```python
from build123d import *

# Parameters (mm, degrees)
SKETCH1_W           = 62.16
SKETCH1_H           = 32.16
SKETCH1_W_2         = 59.16
SKETCH1_H_2         = 29.16
BOSS_EXTRUDE1_DEPTH = 19
SKETCH2_W           = 62.16
SKETCH2_H           = 32.16
BOSS_EXTRUDE2_DEPTH = 1
BOSS_EXTRUDE3_DEPTH = 5
CUT_EXTRUDE4_DEPTH  = 2
CUT_EXTRUDE2_DEPTH  = 33.16
CUT_EXTRUDE3_DEPTH  = 63.16
SKETCH9_W           = 7
SKETCH9_H           = 8.75
CUT_EXTRUDE5_DEPTH  = 63.16


with BuildPart() as part:
    # Sketch1 → Boss-Extrude1 (new body)
    with BuildSketch(Plane.XY):
        Rectangle(SKETCH1_W, SKETCH1_H)
        Rectangle(SKETCH1_W_2, SKETCH1_H_2, mode=Mode.SUBTRACT)
    extrude(amount=BOSS_EXTRUDE1_DEPTH)

    # Sketch2 → Boss-Extrude2 (add)
    with BuildSketch(Plane.XY.offset(19)):
        Rectangle(SKETCH2_W, SKETCH2_H)
    extrude(amount=BOSS_EXTRUDE2_DEPTH)

    # Sketch3 → Boss-Extrude3 (add)
    with BuildSketch(Plane(origin=(0, 0, 0), x_dir=(-1, 0, 0), z_dir=(0, 0, -1))):
        Polygon((-31.08, -16.08), (31.08, -16.08), (31.08, 16.08), (9, 16.08), (-9, 16.08), (-31.08, 16.08), align=None)
        Polygon((29.58, -14.58), (-29.58, -14.58), (-29.58, 14.58), (-9, 14.58), (9, 14.58), (29.58, 14.58), align=None, mode=Mode.SUBTRACT)
    extrude(amount=BOSS_EXTRUDE3_DEPTH)

    # Sketch8 → Cut-Extrude4 (cut, through all)
    with BuildSketch(Plane(origin=(0, 0, 19), x_dir=(-1, 0, 0), z_dir=(0, 0, -1))):
        with BuildLine():
            Line((12, 6.5), (22, 6.5))
            ThreePointArc((22, 6.5), (24, 8.5), (22, 10.5))
            Line((22, 10.5), (12, 10.5))
            ThreePointArc((12, 10.5), (10, 8.5), (12, 6.5))
        make_face()
        with BuildLine():
            Line((12, -2), (22, -2))
            ThreePointArc((22, -2), (24, 0), (22, 2))
            Line((22, 2), (12, 2))
            ThreePointArc((12, 2), (10, 0), (12, -2))
        make_face()
        with BuildLine():
            Line((12, -10.5), (22, -10.5))
            ThreePointArc((22, -10.5), (24, -8.5), (22, -6.5))
            Line((22, -6.5), (12, -6.5))
            ThreePointArc((12, -6.5), (10, -8.5), (12, -10.5))
        make_face()
        with BuildLine():
            Line((-5, -10.5), (5, -10.5))
            ThreePointArc((5, -10.5), (7, -8.5), (5, -6.5))
            Line((5, -6.5), (-5, -6.5))
            ThreePointArc((-5, -6.5), (-7, -8.5), (-5, -10.5))
        make_face()
        with BuildLine():
            Line((-22, -10.5), (-12, -10.5))
            ThreePointArc((-12, -10.5), (-10, -8.5), (-12, -6.5))
            Line((-12, -6.5), (-22, -6.5))
            ThreePointArc((-22, -6.5), (-24, -8.5), (-22, -10.5))
        make_face()
        with BuildLine():
            Line((-22, -2), (-12, -2))
            ThreePointArc((-12, -2), (-10, 0), (-12, 2))
            Line((-12, 2), (-22, 2))
            ThreePointArc((-22, 2), (-24, 0), (-22, -2))
        make_face()
        with BuildLine():
            Line((-5, 6.5), (5, 6.5))
            ThreePointArc((5, 6.5), (7, 8.5), (5, 10.5))
            Line((5, 10.5), (-5, 10.5))
            ThreePointArc((-5, 10.5), (-7, 8.5), (-5, 6.5))
        make_face()
        with BuildLine():
            Line((-22, 6.5), (-12, 6.5))
            ThreePointArc((-12, 6.5), (-10, 8.5), (-12, 10.5))
            Line((-12, 10.5), (-22, 10.5))
            ThreePointArc((-22, 10.5), (-24, 8.5), (-22, 6.5))
        make_face()
        with BuildLine():
            Line((-5, -2), (5, -2))
            ThreePointArc((5, -2), (7, 0), (5, 2))
            Line((5, 2), (-5, 2))
            ThreePointArc((-5, 2), (-7, 0), (-5, -2))
        make_face()
    extrude(amount=-CUT_EXTRUDE4_DEPTH, mode=Mode.SUBTRACT)

    # Sketch5 → Cut-Extrude2 (cut, through all)
    with BuildSketch(Plane(origin=(-15, 16.08, 0), x_dir=(1, 0, 0), z_dir=(0, -1, 0))):
        with BuildLine():
            Line((-9.5, 4), (0.5, 4))
            ThreePointArc((0.5, 4), (2.5, 2), (0.5, 0))
            Line((0.5, 0), (-9.5, 0))
            ThreePointArc((-9.5, 0), (-11.5, 2), (-9.5, 4))
        make_face()
        with BuildLine():
            Line((10, -32.734958022), (20, -32.734958022))
            ThreePointArc((20, -32.734958022), (22, -30.734958022), (20, -28.734958022))
            Line((20, -28.734958022), (10, -28.734958022))
            ThreePointArc((10, -28.734958022), (8, -30.734958022), (10, -32.734958022))
        make_face()
        with BuildLine():
            Line((29.5, -65.469916045), (39.5, -65.469916045))
            ThreePointArc((39.5, -65.469916045), (41.5, -63.469916045), (39.5, -61.469916045))
            Line((39.5, -61.469916045), (29.5, -61.469916045))
            ThreePointArc((29.5, -61.469916045), (27.5, -63.469916045), (29.5, -65.469916045))
        make_face()
        with BuildLine():
            Line((10, -21.734958022), (20, -21.734958022))
            ThreePointArc((20, -21.734958022), (22, -19.734958022), (20, -17.734958022))
            Line((20, -17.734958022), (10, -17.734958022))
            ThreePointArc((10, -17.734958022), (8, -19.734958022), (10, -21.734958022))
        make_face()
        with BuildLine():
            Line((29.5, -54.469916045), (39.5, -54.469916045))
            ThreePointArc((39.5, -54.469916045), (41.5, -52.469916045), (39.5, -50.469916045))
            Line((39.5, -50.469916045), (29.5, -50.469916045))
            ThreePointArc((29.5, -50.469916045), (27.5, -52.469916045), (29.5, -54.469916045))
        make_face()
        with BuildLine():
            Line((-9.5, 11), (0.5, 11))
            ThreePointArc((0.5, 11), (2.5, 13), (0.5, 15))
            Line((0.5, 15), (-9.5, 15))
            ThreePointArc((-9.5, 15), (-11.5, 13), (-9.5, 11))
        make_face()
    extrude(amount=CUT_EXTRUDE2_DEPTH, mode=Mode.SUBTRACT)

    # Sketch7 → Cut-Extrude3 (cut, through all)
    with BuildSketch(Plane(origin=(31.08, -15, 0), x_dir=(0, 0, -1), z_dir=(-1, 0, 0))):
        with BuildLine():
            Line((-15, -26.5), (-15, -19.5))
            ThreePointArc((-15, -19.5), (-13, -17.5), (-11, -19.5))
            Line((-11, -19.5), (-11, -26.5))
            ThreePointArc((-11, -26.5), (-13, -28.5), (-15, -26.5))
        make_face()
        with BuildLine():
            Line((0, -26.5), (0, -19.5))
            ThreePointArc((0, -19.5), (-2, -17.5), (-4, -19.5))
            Line((-4, -19.5), (-4, -26.5))
            ThreePointArc((-4, -26.5), (-2, -28.5), (0, -26.5))
        make_face()
        with BuildLine():
            Line((0, -10.5), (0, -3.5))
            ThreePointArc((0, -3.5), (-2, -1.5), (-4, -3.5))
            Line((-4, -3.5), (-4, -10.5))
            ThreePointArc((-4, -10.5), (-2, -12.5), (0, -10.5))
        make_face()
        with BuildLine():
            Line((-11, -10.5), (-11, -3.5))
            ThreePointArc((-11, -3.5), (-13, -1.5), (-15, -3.5))
            Line((-15, -3.5), (-15, -10.5))
            ThreePointArc((-15, -10.5), (-13, -12.5), (-11, -10.5))
        make_face()
    extrude(amount=CUT_EXTRUDE3_DEPTH, mode=Mode.SUBTRACT)

    # Sketch9 → Cut-Extrude5 (cut, through all)
    with BuildSketch(Plane.ZY.offset(31.08)):
        with Locations((-1.5, 7.875)):
            Rectangle(SKETCH9_W, SKETCH9_H)
        with Locations((-1.5, -7.875)):
            Rectangle(SKETCH9_W, SKETCH9_H)
    extrude(amount=-CUT_EXTRUDE5_DEPTH, mode=Mode.SUBTRACT)


solid = part.part
```
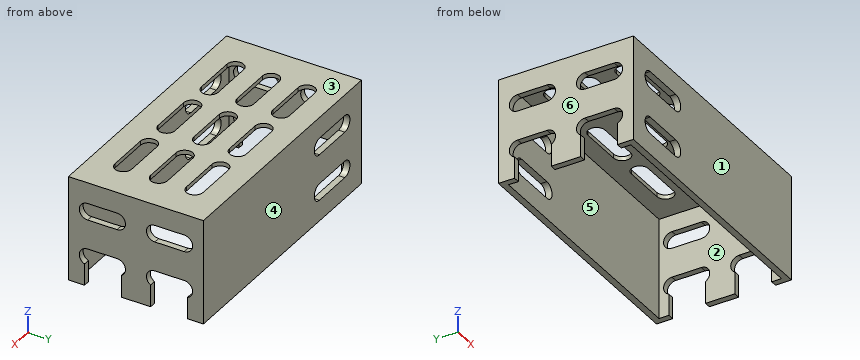
Could you check a few things on this model? Use its own coordinates, in mm. Face numbers are marked on the shaded views. A direction names the side the tool comes from. Coordinates: 2 decimals unless noted, no trailing zeros. Write each loop counter-clockwise with the first axis right and the second up, starting at its lowest first coordinate (ties: lowest second). Pieces come first, ordered by that corner, then holes. Notation, with made-up numbers: M 2,55 L 38,55 A23 cw 38,90 Z; hole C 70,42 d1. An arc over 180 degrees is marked long. Answer as CSV lines item,"result". Start each with the question number.
1) I want a section at C-C, the plane x = 9. Please give me the cut outline in (y, z), and give its area (3 significant figures).
2) For the marked faces 5 and 6, which set-ups out of +Z, -Z, +X, -X, +Y, -Y let a thin tool reach every point of the face, with its end or its side?
3) We'd pull the mould along Y, two halves only. Please class the marked faces 1, 2, 3 and 4: +Y half, -Y half, draft (parallel to the pull), parting line (faces both ways), or undercut.
4) I want a section at B-B, the plane z = 2. Give the number of separate pieces and of enclosed holes in the cut face, and give its area (3 significant figures).
5) For P1, Ø1.2, axis at x = 30.5, y = 9.5, coming from the -Z side; P2, Ø5, axis at x = 18.5, y = 3.5, coming from the -Z side, each with a flat end and sliding along its axis, tell me the tip position at first contact or that it passes through.
6) Please list where these lines run through material, in increasing order: line 1 (X direction, y = 3, z = 5.25); line 2 (Y direction, x = -8, z = 11.5); line 3 (Z direction, x = -0.5, y = 11). Write a range as from..to.
7) I want a section at D-D, the plane y = 8.5. Please give me the cut outline in (x, z).
8) I want a section at A-A, the plane y = 0. Please give me the cut outline in (x, z), and give its area (3 significant figures).
Data:
1,outline,"M -16.08,-5 L -14.58,-5 L -14.58,19 L 14.58,19 L 14.58,-5 L 16.08,-5 L 16.08,20 L -16.08,20 Z"
1,area,"104 mm^2"
2,face 5,"-Z"
2,face 6,"+Z, -Z, -X, +Y, -Y"
3,face 1,"-Y half"
3,face 2,"undercut"
3,face 3,"draft"
3,face 4,"+Y half"
4,separate pieces,"6"
4,enclosed holes,"0"
4,area,"166 mm^2"
5,P1,"stops at z = 4"
5,P2,"stops at z = 19"
6,line 1,"x = -31.08..-29.58, 29.58..31.08"
6,line 2,"y = -16.08..-14.58, 14.58..16.08"
6,line 3,"z = 19..20"
7,outline,"M -31.08,4 L -29.58,4 L -29.58,11 L -31.08,11 Z; M -31.08,15 L -29.58,15 L -29.58,19 L -24,19 L -24,20 L -31.08,20 Z; M -10,19 L -7,19 L -7,20 L -10,20 Z; M 7,19 L 10,19 L 10,20 L 7,20 Z; M 24,19 L 29.58,19 L 29.58,15 L 31.08,15 L 31.08,20 L 24,20 Z; M 29.58,4 L 31.08,4 L 31.08,11 L 29.58,11 Z"
8,outline,"M -31.08,-5 L -29.58,-5 L -29.58,19 L -24,19 L -24,20 L -31.08,20 Z; M -10,19 L -7,19 L -7,20 L -10,20 Z; M 7,19 L 10,19 L 10,20 L 7,20 Z; M 24,19 L 29.58,19 L 29.58,-5 L 31.08,-5 L 31.08,20 L 24,20 Z"
8,area,"92.2 mm^2"
